Work out the finished part from the listing and answer in its coordinate system (mm). A direction names the side the tool comes from. Coordinates: 2 decimals unless noted, no trailing zeros. Loops run counter-clockwise (first coordinate to the right, second up) from the corner with the lowest first, then second, coordinate; pieces in that order, holes last. Notation, with made-up numbers: (-30, 11) - (29, 11) arc R33 ccw to (29, 46) - close; hole circle Ø4 at (62.5, 85.5). An arc over 180 degrees is marked (long way). Write each question's results on one line, items separated by ' | '. Start each with the question number.
1. A cutting plane is placed at C-C on y = 5. Determine the outline of the cut face in (x, z).
2. Each of these flat-tipped pins is pushed along its axis until it touches: P1, Ø4, axis at y = 15, z = 5, coming from the -X side; P2, Ø1.5, axis at y = 16, z = 7, coming from the -X side. Where does it stop, or does it pass through?
3. A cutting plane is placed at A-A on z = 3.5. Determine the outline of the cut face in (x, y), then the cut area to 3 significant figures.
4. Determine the mould class of faces 1 (the cylindrical face through (-1.52, 16.84, 6.69)), 2 (the cylindrical face through (-14.43, 0.6, 4.93)), 3 (the flat face through (-1, 19, 9)), 4 (the flat face through (-14.5, 7, 1)) for opening direction Z: released by +Z, released by -Z, zero draft, split by the parting line, or undercut.
5. Find the intervals of material crossed by line 1 along Z through (x, y) = (-1.8, 15); line 2 along X through (y, z) = (17, 9.25); line 3 along Z through (x, y) = (-1, 12.75), in increasing order. Write a range as [from, to].
6. A cutting plane is placed at D-D on x = -8.5. Determine the outline of the cut face in (y, z), then the cut area to 3 significant figures.
7. A cutting plane is placed at B-B on z = 2.25. Determine the outline of the cut face in (x, y).
8. Which of the six approach directions +Z, -Z, +X, -X, +Y, -Y give full straight-line access (tool end or side, diameter ignored) to faces 5 (the flat face through (-2.6, 7.1, 10)), 6 (the flat face through (-3, 11, 5)), 7 (the flat face through (-14.5, 7, 9))?
from build123d import *

# Parameters (mm, degrees)
F1_DEPTH = 10
F2_SIZE  = 2
F3_R     = 2.5
F4_DEPTH = 25


with BuildPart() as f1:
    # F0 (on Top) → F1 (new body)
    with BuildSketch(Plane.XY):
        with BuildLine():
            ThreePointArc((-2, 0), (-0.585786, 0.585786), (0, 2))
            Line((0, 2), (0, 20))
            Line((0, 20), (-3, 20))
            Line((-3, 20), (-3, 8))
            ThreePointArc((-3, 8), (-8.5, 2.5), (-14, 8))
            Line((-14, 8), (-15, 8))
            Line((-15, 8), (-15, 2))
            ThreePointArc((-15, 2), (-14.414214, 0.585786), (-13, 0))
            Line((-13, 0), (-2, 0))
        make_face()
    extrude(amount=F1_DEPTH)

    # F2
    f2_edges = [f1.edges().sort_by_distance(p)[0] for p in [
        (-1.5, 20, 10),
        (-1.5, 20, 0),
        (-14.5, 8, 10),
        (-14.5, 8, 0),
    ]]
    chamfer(f2_edges, length=F2_SIZE)

    # F3 (on face) → F4 (cut)
    with BuildSketch(Plane(origin=(-3, 0, 0), x_dir=(0, -1, 0), z_dir=(-1, 0, 0))):
        with Locations((-15, 5)):
            Circle(F3_R)
    extrude(amount=-F4_DEPTH, mode=Mode.SUBTRACT)


solid = f1.part
Values:
1) outline: (-15, 0) - (-13.11, 0) - (-13.11, 10) - (-15, 10) - close; (-3.89, 0) - (0, 0) - (0, 10) - (-3.89, 10) - close
2) P1: through | P2: x = -3
3) outline: (-15, 2) arc R2 ccw to (-13, 0) - (-2, 0) arc R2 ccw to (0, 2) - (0, 13) - (-3, 13) - (-3, 8) arc R5.5 cw to (-14, 8) - (-15, 8) - close; (-3, 17) - (0, 17) - (0, 20) - (-3, 20) - close | area: 94.8 mm^2
4) face 1: undercut | face 2: zero draft | face 3: released by +Z | face 4: released by -Z
5) line 1: [0, 2.5], [7.5, 10] | line 2: [-3, 0] | line 3: [0, 3.91], [6.09, 10]
6) outline: (0, 0) - (2.5, 0) - (2.5, 10) - (0, 10) - close | area: 25.0 mm^2
7) outline: (-15, 2) arc R2 ccw to (-13, 0) - (-2, 0) arc R2 ccw to (0, 2) - (0, 20) - (-3, 20) - (-3, 8) arc R5.5 cw to (-14, 8) - (-15, 8) - close
8) face 5: +Z, +X, -X, +Y, -Y | face 6: +Z, -Z, -X, +Y | face 7: +Z, -X, +Y
